Can you work these out from the model? Positions are in its coordinate system, mm. A direction names the side the tool comes from. Give positions to 0.01 mm unless a question says otherwise; leave off trailing zeros. Loops run counter-clockwise (first coordinate to the right, second up) from the corner with the lowest first, then second, coordinate; pieces in that order, holes last. Notation, with made-up numbers: M 40,-10 L 64,-10 A32 cw 64,16 Z; hole C 84.25,4 d4. An arc over 180 degrees is marked long. Use CSV: the item, a comma, the result in double quotes.
from build123d import *

# Parameters (mm, degrees)
SKETCH1_W           = 25.4
SKETCH1_H           = 50.8
SKETCH1_W_2         = 19.05
SKETCH1_H_2         = 44.45
BOSS_EXTRUDE1_DEPTH = 685.8
SKETCH2_R           = 3.175
SKETCH2_R_2         = 2.38125
CUT_EXTRUDE1_DEPTH  = 688.796168934
SKETCH3_R           = 2.38125
CUT_EXTRUDE2_DEPTH  = 3.175
SKETCH4_R           = 2.38125
CUT_EXTRUDE3_DEPTH  = 688.796168934


with BuildPart() as part:
    # Sketch1 → Boss-Extrude1 (new body)
    with BuildSketch(Plane.XY):
        Rectangle(SKETCH1_W, SKETCH1_H)
        Rectangle(SKETCH1_W_2, SKETCH1_H_2, mode=Mode.SUBTRACT)
    extrude(amount=BOSS_EXTRUDE1_DEPTH)

    # Sketch2 → Cut-Extrude1 (cut, through all)
    with BuildSketch(Plane(origin=(0, 25.4, 0), x_dir=(1, 0, 0), z_dir=(0, 1, 0))):
        with Locations(Location((0, -12.7, 0), (0, 0, 270))):
            Circle(SKETCH2_R)
        with Locations(Location((0, -151.012144, 0), (0, 0, 270))):
            Circle(SKETCH2_R)
        with Locations((0, -534.787856)):
            Circle(SKETCH2_R)
        with Locations((0, -673.1)):
            Circle(SKETCH2_R)
        with Locations(Location((0, -185.1062846, 0), (0, 0, 270))):
            Circle(SKETCH2_R_2)
        with Locations(Location((0, -197.8062846, 0), (0, 0, 270))):
            Circle(SKETCH2_R_2)
        with Locations(Location((0, -210.5062846, 0), (0, 0, 270))):
            Circle(SKETCH2_R_2)
        with Locations(Location((0, -223.2062846, 0), (0, 0, 270))):
            Circle(SKETCH2_R_2)
        with Locations(Location((0, -235.9062846, 0), (0, 0, 270))):
            Circle(SKETCH2_R_2)
        with Locations((0, -449.8937154)):
            Circle(SKETCH2_R_2)
        with Locations((0, -462.5937154)):
            Circle(SKETCH2_R_2)
        with Locations((0, -475.2937154)):
            Circle(SKETCH2_R_2)
        with Locations((0, -487.9937154)):
            Circle(SKETCH2_R_2)
        with Locations((0, -500.6937154)):
            Circle(SKETCH2_R_2)
    extrude(amount=-CUT_EXTRUDE1_DEPTH, mode=Mode.SUBTRACT)

    # Sketch3 → Cut-Extrude2 (cut)
    with BuildSketch(Plane(origin=(12.7, 0, 0), x_dir=(0, 0, -1), z_dir=(1, 0, 0))):
        with Locations((-361.95, -12.7)):
            Circle(SKETCH3_R)
        with Locations((-342.9, -12.7)):
            Circle(SKETCH3_R)
        with Locations(Location((-323.85, -12.7, 0), (0, 0, 180))):
            Circle(SKETCH3_R)
        with Locations((-323.85, 12.7)):
            Circle(SKETCH3_R)
        with Locations(Location((-361.95, 12.7, 0), (0, 0, 180))):
            Circle(SKETCH3_R)
        with Locations(Location((-342.9, 12.7, 0), (0, 0, 180))):
            Circle(SKETCH3_R)
    extrude(amount=-CUT_EXTRUDE2_DEPTH, mode=Mode.SUBTRACT)

    # Sketch4 → Cut-Extrude3 (cut, through all)
    with BuildSketch(Plane(origin=(0, -25.4, 0), x_dir=(-1, 0, 0), z_dir=(0, -1, 0))):
        with Locations(Location((0, -342.9, 0), (0, 0, 90))):
            Circle(SKETCH4_R)
        with Locations(Location((0, -361.95, 0), (0, 0, 90))):
            Circle(SKETCH4_R)
        with Locations(Location((0, -323.85, 0), (0, 0, 180))):
            Circle(SKETCH4_R)
    extrude(amount=-CUT_EXTRUDE3_DEPTH, mode=Mode.SUBTRACT)


solid = part.part
Q1. If we mould it in two halves opening along X, with no side actions, what happens to faces 3 (the flat face through (-12.7, 0, 338)), 4 (the flat face through (0, -25.4, 338)), 5 (the flat face through (12.7, 0, 338)), 6 (the flat face through (0, -22.225, 338))? For each: released by +X, released by -X, zero draft, split by the parting line, or undercut.
Model answer:
face 3,"released by -X"
face 4,"zero draft"
face 5,"released by +X"
face 6,"undercut"
Q2. I want a section at A-A, the plane y = 0.5. Please give me the cut outline in (x, z) (3 decimals).
Model answer:
outline,"M -12.7,0 L -9.525,0 L -9.525,685.8 L -12.7,685.8 Z; M 9.525,0 L 12.7,0 L 12.7,685.8 L 9.525,685.8 Z"
Q3. I want a section at B-B, the plane z = 414. Please give me the cut outline in (x, y) (3 decimals).
Model answer:
outline,"M -12.7,-25.4 L 12.7,-25.4 L 12.7,25.4 L -12.7,25.4 Z; hole M -9.525,-22.225 L 9.525,-22.225 L 9.525,22.225 L -9.525,22.225 Z"
Q4. I'm going to push a flat-ended pin straight in: P1, Ø3, axis at y = 12.7, z = 361.95, coming from the +X side (3 decimals). Where does the tip first touch, or does it pass through?
Model answer:
P1,"x = -9.525"
Q5. Please list where these lines run through material, in increasing order: L1, parallel to Y at x = 4, z = 571 (3 decimals); L2, parallel to X at y = -21, z = 596.5 (3 decimals); L3, parallel to X at y = 23, z = 361. Write a range as from..to.
Model answer:
L1,"-25.4..-22.225, 22.225..25.4"
L2,"-12.7..-9.525, 9.525..12.7"
L3,"-12.7..-2.18, 2.18..12.7"
Q6. For faces 1 (the flat face through (-10, -2, 685.8)), 2 (the flat face through (9.525, 0, 338)), which set-ups out of +Z, -Z, +X, -X, +Y, -Y let a thin tool reach every point of the face, with its end or its side?
Model answer:
face 1,"+Z, +X, -X, +Y, -Y"
face 2,"+Z, -Z"
